Geometry check sheet. Reference: the model listing, model coordinates, mm. Coordinates: 2 decimals unless noted, no trailing zeros. Loops run counter-clockwise (first coordinate to the right, second up) from the corner with the lowest first, then second, coordinate; pieces in that order, holes last. Notation, with made-up numbers: (40, 73) - (59, 73) arc R17 ccw to (59, 88) - close; hole circle Ø9 at (-24, 80.5). An arc over 180 degrees is marked (long way). Write item = value, one per line. Start each with the question number.
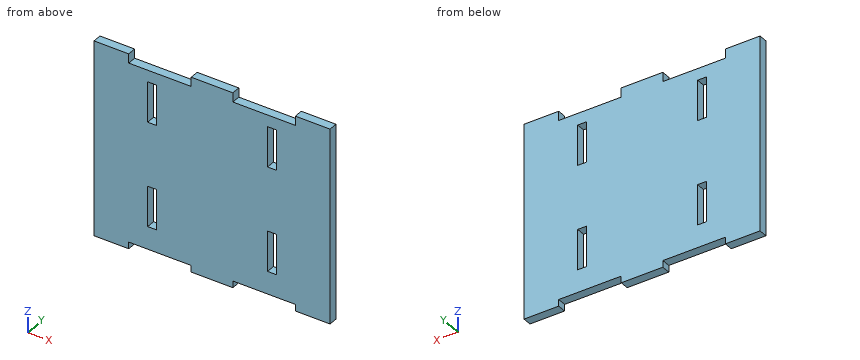
from build123d import *

# Parameters (mm, degrees)
SKETCH1_W           = 85
SKETCH1_H           = 70
BOSS_EXTRUDE1_DEPTH = 3.175
SKETCH2_W           = 3.175
SKETCH2_H           = 14.492
SKETCH2_W_2         = 22.5
SKETCH2_H_2         = 2.38125
SKETCH2_H_3         = 3.313043478
CUT_EXTRUDE1_DEPTH  = 4.175


with BuildPart() as part:
    # Sketch1 → Boss-Extrude1 (new body)
    with BuildSketch(Plane(origin=(0, 0, 0), x_dir=(1, 0, 0), z_dir=(0, 1, 0))):
        with Locations((42.5, 35)):
            Rectangle(SKETCH1_W, SKETCH1_H)
    extrude(amount=BOSS_EXTRUDE1_DEPTH)

    # Sketch2 → Cut-Extrude1 (cut, through all)
    with BuildSketch(Plane.XZ):
        with Locations((20.9125, -14.746)):
            Rectangle(SKETCH2_W, SKETCH2_H)
        with Locations((20.9125, -52.246)):
            Rectangle(SKETCH2_W, SKETCH2_H)
        with Locations((64.0875, -14.746)):
            Rectangle(SKETCH2_W, SKETCH2_H)
        with Locations((64.0875, -52.246)):
            Rectangle(SKETCH2_W, SKETCH2_H)
        with Locations((61.25, -68.809375)):
            Rectangle(SKETCH2_W_2, SKETCH2_H_2)
        with Locations((23.75, -68.809375)):
            Rectangle(SKETCH2_W_2, SKETCH2_H_2)
        with Locations((61.25, -1.656521739)):
            Rectangle(SKETCH2_W_2, SKETCH2_H_3)
        with Locations((23.75, -1.656521739)):
            Rectangle(SKETCH2_W_2, SKETCH2_H_3)
    extrude(amount=-CUT_EXTRUDE1_DEPTH, mode=Mode.SUBTRACT)


solid = part.part
(1) Scan lines: line 1 (X direction, y = 3, z = -49.5) (3 decimals); line 2 (Z direction, x = 21.5, y = 2.85); line 3 (X direction, y = 0.65, z = -3). Record each from-to range of solid material in increasing order.
(2) Depth check by flat-ended pin: pin 1 (1.6 mm diameter, centred on x = 24.5, y = 2, fed in from -Z); pin 2 (1 mm diameter, centred on x = 56.5, y = 1.5, fed in from +Z); pin 3 (2 mm diameter, centred on x = 28, z = -55.5, fed in from -Y). Enter the tip coordinate at first touch or a pass-through.
(3) Sectioned sample at A-A on z = -10.5. Enter the section's corners in (x, y) (3 decimals), plus the area to 3 significant figures.
(4) Sectioned sample at C-C on y = 1.35. Count the separate pieces of the cut face and the enclosed holes in it, plus the area to 3 significant figures.
(5) Sectioned sample at B-B on x = 33. Enter the section's corners in (y, z) (3 decimals), plus the area to 3 significant figures.
Working result:
q1.line_1 = 0 to 19.325, 22.5 to 62.5, 65.675 to 85
q1.line_2 = -67.62 to -59.49, -45 to -21.99, -7.5 to -3.31
q1.line_3 = 0 to 12.5, 35 to 50, 72.5 to 85
q2.pin_1 = -67.62
q2.pin_2 = -3.31
q2.pin_3 = 0
q3.outline = (0, 0) - (19.325, 0) - (19.325, 3.175) - (0, 3.175) - close; (22.5, 0) - (62.5, 0) - (62.5, 3.175) - (22.5, 3.175) - close; (65.675, 0) - (85, 0) - (85, 3.175) - (65.675, 3.175) - close
q3.area = 250 mm2
q4.separate_pieces = 1
q4.enclosed_holes = 4
q4.area = 5,510 mm2
q5.outline = (0, -67.619) - (3.175, -67.619) - (3.175, -3.313) - (0, -3.313) - close
q5.area = 204 mm2
